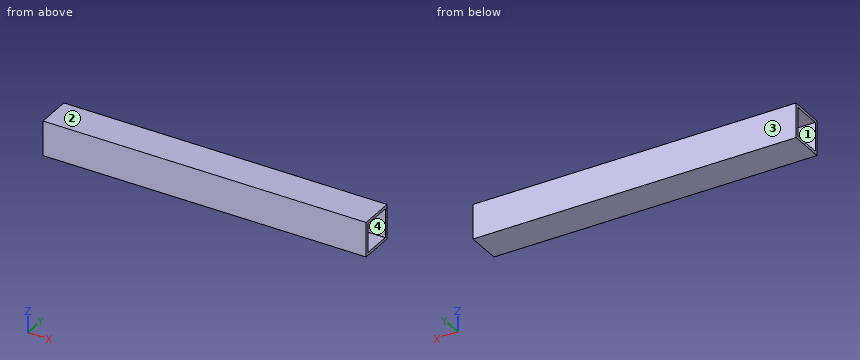
from build123d import *

# Parameters (mm, degrees)
SKETCH1_W           = 19.05
SKETCH1_H           = 19.05
SKETCH1_W_2         = 15.875
SKETCH1_H_2         = 15.875
BOSS_EXTRUDE1_DEPTH = 88.9


with BuildPart() as part:
    # Sketch1 → Boss-Extrude1 (new body, symmetric)
    with BuildSketch(Plane(origin=(0, 0, 0), x_dir=(0, -1, 0), z_dir=(1, 0, 0))):
        Rectangle(SKETCH1_W, SKETCH1_H)
        Rectangle(SKETCH1_W_2, SKETCH1_H_2, mode=Mode.SUBTRACT)
    extrude(amount=BOSS_EXTRUDE1_DEPTH, both=True)


solid = part.part
Design review of the part built by this model. Coordinates are the model's own, in mm. Face numbers are marked on the shaded views. Coordinates: 2 decimals unless noted, no trailing zeros. Loops run counter-clockwise (first coordinate to the right, second up) from the corner with the lowest first, then second, coordinate; pieces in that order, holes last. Notation, with made-up numbers: M -24.5,5.5 L 27.5,5.5 A12 ccw 27.5,21.5 Z; hole C 62,11 d5. An arc over 180 degrees is marked long. Use one line per item in the form item = value.
(1) Consider section B-B (y = 3.25). Write out the cut boundary in (x, z) (1 decimal).
Return value:
outline = M -88.9,-9.5 L 88.9,-9.5 L 88.9,-7.9 L -88.9,-7.9 Z; M -88.9,7.9 L 88.9,7.9 L 88.9,9.5 L -88.9,9.5 Z
(2) Draft analysis for pull direction Z (two halves, no side actions). For the marked faces 1, 2, 3 and 4, state which applies: pulls with the +Z half, pulls with the -Z half, needs draft (parallel to the pull), parting line crosses it, or undercut.
Return value:
face_1 = undercut
face_2 = pulls with the +Z half
face_3 = needs draft
face_4 = undercut
(3) For line 1 along Y through (x, z) = (-12.5, -2.5) (1 decimal), list the stretches that pass through material, from the lowest coordinate up. Write a range as from..to.
Return value:
line_1 = -9.5..-7.9, 7.9..9.5
(4) Clearance check with a flat-ended pin moving along its axis: P1, Ø1, axis at y = 3.5, z = -7.5, coming from the +X side. State where the tip first meets the part, or that it passes through.
Return value:
P1 = 88.9
(5) Consider section A-A (x = 22). Write out the cut boundary in (y, z) (1 decimal).
Return value:
outline = M -9.5,-9.5 L 9.5,-9.5 L 9.5,9.5 L -9.5,9.5 Z; hole M -7.9,-7.9 L 7.9,-7.9 L 7.9,7.9 L -7.9,7.9 Z
